from build123d import *

# Parameters (mm, degrees)
SALIENTE_EXTRUIR1_DEPTH = 10
CROQUIS2_R              = 2.5
CORTAR_EXTRUIR1_DEPTH   = 10
REDONDEO1_R             = 4


with BuildPart() as part:
    # Croquis1 → Saliente-Extruir1 (new body)
    with BuildSketch(Plane(origin=(0, 0, 0), x_dir=(1, 0, 0), z_dir=(0, 1, 0))):
        with BuildLine():
            Line((-1, 34.985711369), (-1, 46.834087473))
            Line((-1, 46.834087473), (-3.5, 46.834087473))
            Line((-3.5, 46.834087473), (-3.5, 36.834087473))
            ThreePointArc((-3.5, 36.834087473), (0, -37), (3.5, 36.834087473))
            Line((3.5, 36.834087473), (3.5, 46.834087473))
            Line((3.5, 46.834087473), (1, 46.834087473))
            Line((1, 46.834087473), (1, 34.985711369))
            ThreePointArc((1, 34.985711369), (0, -35), (-1, 34.985711369))
        make_face()
    extrude(amount=SALIENTE_EXTRUIR1_DEPTH)

    # Croquis2 → Cortar-Extruir1 (cut)
    with BuildSketch(Plane.ZY.offset(3.5)):
        with Locations((-41.834087473, 5)):
            Circle(CROQUIS2_R)
    extrude(amount=-CORTAR_EXTRUIR1_DEPTH, mode=Mode.SUBTRACT)

    # Redondeo1
    redondeo1_edges = [part.edges().sort_by_distance(p)[0] for p in [
        (-2.25, 0, -46.834087473),
        (-2.25, 10, -46.834087473),
        (2.25, 10, -46.834087473),
        (2.25, 0, -46.834087473),
    ]]
    fillet(redondeo1_edges, radius=REDONDEO1_R)


solid = part.part
Source: CAD feature listing. Evaluate the final solid. Frame: model axes, mm. A direction names the side the tool comes from. Give positions to 0.01 mm unless a question says otherwise; leave off trailing zeros. Order: outer loops, then holes, each group sorted by start corner. A loop starts at its lowest first (then second) coordinate and runs counter-clockwise, first axis right, second up. Notation, with made-up numbers: (33, -9) -> (74, -9) arc R26 ccw to (74, 16) -> close; hole circle Ø10 at (81.25, -6). An arc over 180 degrees is marked (long way). Write item = value, one per line.
Item 1: Mould query, pull axis X, two halves, no side actions, for faces 4 (the face through (-2, 5, -46.834)), 5 (the face through (3.5, 3, -40)), 6 (the face through (1, 5, -38)). Classes: +X half, -X half, draft (parallel to the pull), parting line (faces both ways), or undercut.
Check result:
face_4 = draft
face_5 = +X half
face_6 = undercut
Item 2: Section query C-C (x = -18.5). Output: boundary loops of the cut face in (y, z), then the cut area to 3 significant figures.
Check result:
outline = (0, -32.04) -> (10, -32.04) -> (10, -29.71) -> (0, -29.71) -> close; (0, 29.71) -> (10, 29.71) -> (10, 32.04) -> (0, 32.04) -> close
area = 46.6 mm²
Item 3: Section query B-B (y = 5). Output: boundary loops of the cut face in (x, z).
Check result:
outline = (-3.5, -46.83) -> (-1, -46.83) -> (-1, -44.33) -> (-3.5, -44.33) -> close; (-3.5, -39.33) -> (-1, -39.33) -> (-1, -34.99) arc R35 cw (long way) to (1, -34.99) -> (1, -39.33) -> (3.5, -39.33) -> (3.5, -36.83) arc R37 ccw (long way) to (-3.5, -36.83) -> close; (1, -46.83) -> (3.5, -46.83) -> (3.5, -44.33) -> (1, -44.33) -> close
Item 4: Contact query for flat-ended pins moving along their axis: pin 1 (6 mm diameter, centred on y = 5, z = -41.83, fed in from +X); pin 2 (3 mm diameter, centred on y = 6, z = 7, fed in from +X); pin 3 (1.5 mm diameter, centred on y = 5, z = -7, fed in from -X). Output: stop coordinate, or through.
Check result:
pin_1 = 3.5
pin_2 = 36.59
pin_3 = -36.47
Item 5: Ray query, probe 1 along X at (y, z) = (8.5, -38); probe 2 along X at (y, z) = (6.5, 0); probe 3 along Z at (x, y) = (-8, 3.25). Return the intervals inside material, ascending.
Check result:
probe_1 = -3.5 to -1, 1 to 3.5
probe_2 = -37 to -35, 35 to 37
probe_3 = -36.12 to -34.07, 34.07 to 36.12
Item 6: Section query D-D (x = -2). Output: boundary loops of the cut face in (y, z), then the cut area to 3 significant figures.
Check result:
outline = (0, -42.83) arc R4 ccw to (4, -46.83) -> (6, -46.83) arc R4 ccw to (10, -42.83) -> (10, -34.94) -> (0, -34.94) -> close; (0, 34.94) -> (10, 34.94) -> (10, 36.95) -> (0, 36.95) -> close; hole circle Ø5 at (5, -41.83)
area = 112 mm²
Item 7: Section query A-A (z = 0). Output: boundary loops of the cut face in (x, y).
Check result:
outline = (-37, 0) -> (-35, 0) -> (-35, 10) -> (-37, 10) -> close; (35, 0) -> (37, 0) -> (37, 10) -> (35, 10) -> close
Item 8: Set-up query: faces 1 (the face through (-2.27, 1.14, -45.63)), 2 (the face through (-3.5, 3, -40)), 3 (the face through (-1, 5, -38)). Return all of +Z, -Z, +X, -X, +Y, -Y with unobstructed straight access to the full face (end or side cutting, diameter ignored); none if empty.
Check result:
face_1 = -Z, +X, -X, -Y
face_2 = -Z, -X, +Y, -Y
face_3 = -Z, +Y, -Y
